```python
from build123d import *

# Parameters (mm, degrees)
F0_R     = 35.8722677543
F1_DEPTH = 3.048


with BuildPart() as f1:
    # F0 (on Front) → F1 (new body)
    with BuildSketch(Plane.XZ):
        with Locations((-16.5389925241, 0)):
            Circle(F0_R)
        with BuildLine():
            Line((-7.0172841661, -16.8818086386), (-16.4545532316, -24.4767442346))
            add(Edge.make_bspline(
                [(-16.4545532316, -24.4767442346), (-16.8368068171, -24.1939949846), (-17.6591396418, -23.5857234125), (-19.1498410611, -22.2695343414), (-20.1683555608, -20.6216308858), (-21.0775722167, -18.8965393574), (-21.4159472056, -17.0038620995), (-21.7830891286, -15.1529140615), (-21.7468870372, -14.4858724729), (-21.7320397496, -14.2123037949)],
                knots=[0, 0, 0, 0, 0.1335803654, 0.2873681853, 0.4404495382, 0.5922340471, 0.7460919747, 0.8958666386, 1, 1, 1, 1], degree=3))
            Line((-21.7320397496, -14.2123037949), (-21.7320397496, 3.0830921605))
            add(Edge.make_bspline(
                [(-25.3525003791, 6.3037872314), (-25.0035694122, 6.4840549077), (-24.4211323439, 6.784958487), (-23.9671240009, 6.9548534074), (-23.2729776472, 6.9757200424), (-22.5775088209, 6.5504818074), (-22.1244270369, 6.173485954), (-21.610740531, 4.6481096322), (-21.6911569949, 3.6105665011), (-21.7320397496, 3.0830921605)],
                knots=[0, 0, 0, 0, 0.1543245572, 0.2575992135, 0.3790212722, 0.5114796991, 0.6251869619, 0.8094495986, 1, 1, 1, 1], degree=3))
            add(Edge.make_bspline(
                [(-25.499086827, 6.6551566124), (-25.6385246281, 6.5602763851), (-25.8639647367, 6.4068760261), (-25.8485920944, 6.1900064814), (-25.7133319129, 6.107920989), (-25.4915746658, 6.2047990872), (-25.3967399547, 6.2722990707), (-25.3525003791, 6.3037872314)],
                knots=[0, 0, 0, 0, 0.2846359539, 0.4601934329, 0.6140274626, 0.8199471371, 1, 1, 1, 1], degree=3))
            Line((-25.499086827, 6.6551566124), (-16.7787857354, 13.7423193082))
            Line((-16.7787857354, 13.7423193082), (-15.3459142894, 12.4895032495))
            Line((-15.3459142894, 12.4895032495), (-12.911436148, 10.0866425782))
            Line((-12.911436148, 10.0866425782), (-11.1092906445, 8.6638955399))
            Line((-11.1092906445, 8.6638955399), (-9.5916930586, 7.6521639712))
            add(Edge.make_bspline(
                [(-9.5916930586, 7.6521639712), (-9.349729434, 7.5241534863), (-8.901127436, 7.2868212866), (-8.2178516893, 7.2340472433), (-8.2081308902, 6.9188765434), (-8.3758976081, 6.7811977964), (-8.7490682058, 6.8679608418), (-9.3993086232, 6.7593583892), (-9.9663047763, 6.4823224185), (-10.5756488537, 6.11491138), (-11.205548345, 5.5589280964), (-11.5528638282, 4.9166655347), (-11.7238497245, 4.3198587863), (-11.8153616786, 4.0004467592)],
                knots=[0, 0, 0, 0, 0.1084812333, 0.2011248513, 0.256700979, 0.3067833697, 0.3784833865, 0.4755646116, 0.5711165511, 0.6723420327, 0.7810491113, 0.8828170972, 1, 1, 1, 1], degree=3))
            Line((-11.8153616786, 4.0004467592), (-11.8153616786, 0))
            Line((-11.8153616786, 0), (-11.8153616786, -9.1262217611))
            Line((-11.8153616786, -9.1262217611), (-11.8153616786, -14.9436760694))
            add(Edge.make_bspline(
                [(-11.8153616786, -14.9436760694), (-11.752930028, -15.2417605806), (-11.6349053575, -15.8052780581), (-11.1592093747, -16.3296727482), (-10.6540369389, -16.9123160957), (-9.9771466257, -17.3074550788), (-9.2864785852, -17.4372864271), (-8.2735107194, -17.4033083883), (-7.8177957528, -17.3297418503), (-7.3118112692, -17.0466138374), (-7.0172841661, -16.8818086386)],
                knots=[0, 0, 0, 0, 0.1334555489, 0.25229266, 0.3778349348, 0.5020083005, 0.6239272043, 0.7656469646, 0.8635860924, 1, 1, 1, 1], degree=3))
        make_face(mode=Mode.SUBTRACT)
        with BuildLine():
            add(Edge.make_bspline(
                [(-16.5393147618, 16.0637069494), (-16.0952406112, 16.3723268092), (-15.1531884741, 17.0270282778), (-13.4519795924, 18.3410565916), (-12.307992004, 19.2477362645), (-11.7960339961, 20.2438380114), (-11.5315010771, 20.7585319877)],
                knots=[0, 0, 0, 0, 0.2477515115, 0.5255762818, 0.7548613575, 1, 1, 1, 1], degree=3))
            add(Edge.make_bspline(
                [(-11.5315010771, 20.7585319877), (-11.3886353445, 21.131794299), (-11.0776192325, 21.9443795897), (-11.422463862, 23.7306869337), (-12.2198755022, 24.6869108683), (-13.0056152853, 25.8167281527), (-14.8153986013, 26.8110341086), (-16.3083312279, 26.5741886558), (-17.7349189872, 26.6068206692), (-19.3878002125, 25.774154561), (-20.5117985183, 24.2148361341), (-21.1179317123, 22.375294743), (-20.7808520416, 20.7288316555), (-19.8509306492, 19.0194517847), (-18.4767807189, 17.9221470779), (-17.54650896, 16.6853845369), (-16.8593317149, 16.2612332732), (-16.5393147618, 16.0637069494)],
                knots=[0, 0, 0, 0, 0.0591766629, 0.1288265232, 0.1875414136, 0.2494013304, 0.3235814023, 0.3879482515, 0.4504797153, 0.5207736845, 0.5940792329, 0.6664881359, 0.7341792345, 0.8072636763, 0.8777722528, 0.9430788032, 1, 1, 1, 1], degree=3))
        make_face(mode=Mode.SUBTRACT)
    extrude(amount=F1_DEPTH)


solid = f1.part
```
Geometry: final body of the model. Coordinates: model frame, mm. A direction names the side the tool comes from. Coordinates: 2 decimals unless noted, no trailing zeros. Order: outer loops, then holes, each group sorted by start corner. A loop starts at its lowest first (then second) coordinate and runs counter-clockwise, first axis right, second up. Notation, with made-up numbers: (-19.5, 80) - (1.5, 80) arc R9 ccw to (1.5, 94) - close; hole circle Ø3 at (33, 77). An arc over 180 degrees is marked (long way). Return JSON: item names as keys, results as strings. Group by question number.
1. Cut plane C-C (y = -2.4). Count the separate pieces of the cut face and the enclosed holes in it, plus the area to 3 significant figures.
2. Cut plane A-A (z = -9). Output: boundary loops of the cut face in (x, y).
3. Cut plane B-B (z = 0). Output: boundary loops of the cut face in (x, y), plus the area to 3 significant figures.
4. Material intervals for line 1 along Z through (x, y) = (-14.5, -1.7); line 2 along Z through (x, y) = (-19.5, -0.8); line 3 along X through (y, z) = (-0.4, -9.5), sorted ascending. Write a range as [from, to].
5. Set-up query: faces 1 (the face through (-9, 0, 1)), 2 (the face through (-12.023, -1.503, 9.385)). Return all of +Z, -Z, +X, -X, +Y, -Y with unobstructed straight access to the full face (end or side cutting, diameter ignored); none if empty.
6. Cut plane D-D (x = -2). Output: boundary loops of the cut face in (y, z).
7. Pull-direction query (X, two-part tool) for faces 3 (the face through (-9, -3.048, 1)), 4 (the face through (-11.815, -2, -5)), 5 (the face through (17.677, -1.503, 10.775)); classes: pulls with the +X half, pulls with the -X half, needs draft (parallel to the pull), parting line crosses it, or undercut.
Resolved:
{
 "1": {"separate pieces": "1", "enclosed holes": "2", "area": "3,610 mm²"},
 "2": {"outline": "(-51.26, -3.05) - (-21.73, -3.05) - (-21.73, 0) - (-51.26, 0) - close; (-11.82, -3.05) - (18.19, -3.05) - (18.19, 0) - (-11.82, 0) - close"},
 "3": {"outline": "(-52.41, -3.05) - (-21.73, -3.05) - (-21.73, 0) - (-52.41, 0) - close; (-11.82, -3.05) - (19.33, -3.05) - (19.33, 0) - (-11.82, 0) - close", "area": "188 mm²"},
 "4": {"line 1": "z = [-35.81, -22.9], [11.65, 17.54], [26.52, 35.81]", "line 2": "z = [-35.75, -21.65], [11.53, 18.82], [25.46, 35.75]", "line 3": "x = [-51.13, -21.73], [-11.82, 18.05]"},
 "5": {"face 1": "+Z, -Z, +X, -X, +Y", "face 2": "+Y, -Y"},
 "6": {"outline": "(-3.05, -32.79) - (0, -32.79) - (0, 32.79) - (-3.05, 32.79) - close"},
 "7": {"face 3": "needs draft", "face 4": "undercut", "face 5": "parting line crosses it"}
}
